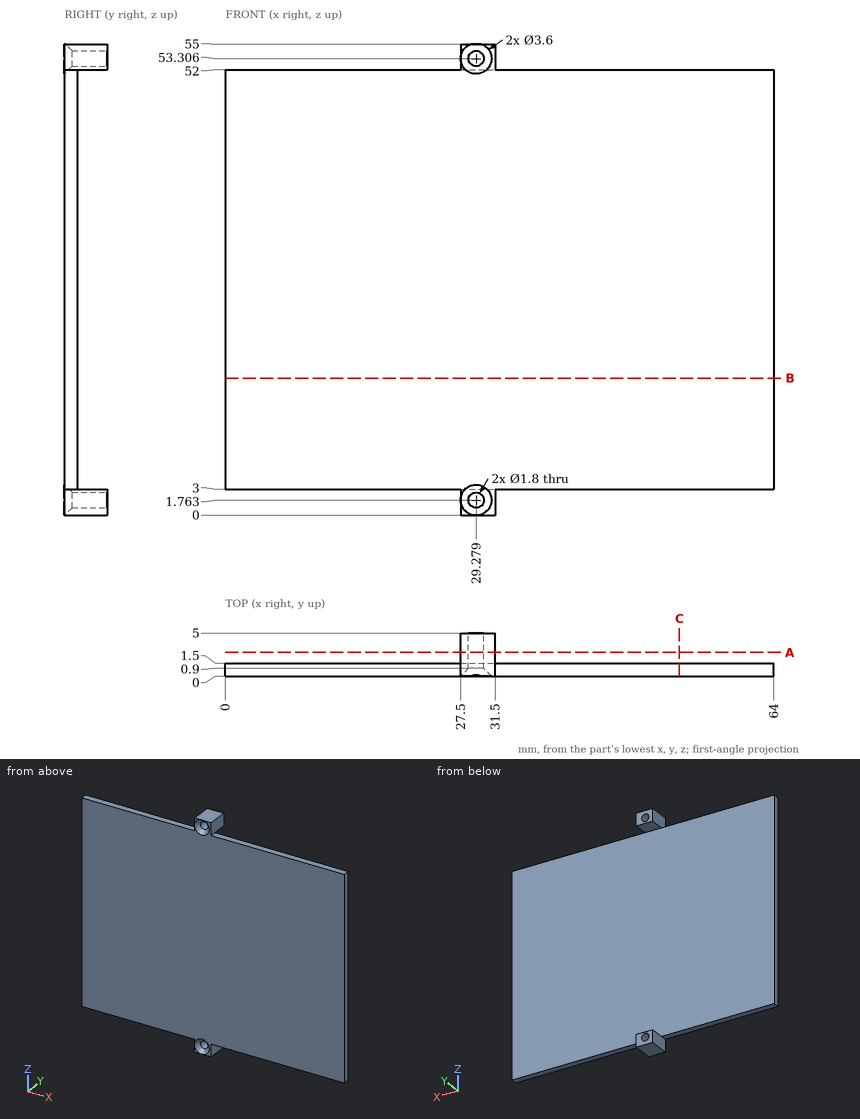
Source: three-view drawing plus pictorial views. Frame: mm from the lowest corner of the part. Give positions to 0.01 mm unless a question says otherwise; leave off trailing zeros. Order: outer loops, then holes, each group sorted by start corner. A loop starts at its lowest first (then second) coordinate and runs counter-clockwise, first axis right, second up. Notation, with made-up numbers: (87, 49.25) -> (141, 49.25) arc R27 cw to (141, 70.25) -> close; hole circle Ø11 at (29.5, 20.5). An arc over 180 degrees is marked (long way). Put each result on its own line as item: value.
Q1. Material intervals for L1, parallel to Z at x = 28.5, y = 2.15 (1 decimal); L2, parallel to Y at x = 18.5, z = 45; L3, parallel to Z at x = 32, y = 1.2, sorted ascending.
Here are the results:
L1: z = 0 to 1.3, 2.2 to 3, 52 to 52.9, 53.8 to 55
L2: y = 0 to 1.5
L3: z = 3 to 52
Q2. Section C-C, the plane x = 53. Return loops of the section in (y, z).
Here are the results:
outline: (0, 3) -> (1.5, 3) -> (1.5, 52) -> (0, 52) -> close
Q3. Section B-B, the plane z = 16. Return loops of the section in (x, y).
Here are the results:
outline: (0, 0) -> (64, 0) -> (64, 1.5) -> (0, 1.5) -> close
Q4. Pin query (flat end, axial travel): pin 1 (1.6 mm diameter, centred on x = 40.5, y = 0.5, fed in from +Z); pin 2 (0.8 mm diameter, centred on x = 55.5, y = 0.5, fed in from -Z); pin 3 (1.6 mm diameter, centred on x = 29.28, z = 53.31, fed in from -Y); pin 4 (2.5 mm diameter, centred on y = 3, z = 1.5, fed in from -X). Return the tip coordinate at first contact, or that it passes through.
Here are the results:
pin 1: stops at z = 52
pin 2: stops at z = 3
pin 3: passes through
pin 4: stops at x = 27.5
Q5. Section A-A, the plane y = 2.75. Return loops of the section in (x, z), then the cut area to 3 significant figures.
Here are the results:
outline: (27.5, 0) -> (31.5, 0) -> (31.5, 3) -> (27.5, 3) -> close; (27.5, 52) -> (31.5, 52) -> (31.5, 55) -> (27.5, 55) -> close; hole circle Ø1.8 at (29.28, 1.76); hole circle Ø1.8 at (29.28, 53.31)
area: 18.9 mm^2
